Design review of the part built by this model. Coordinates are the model's own, in mm. A direction names the side the tool comes from. Coordinates: 2 decimals unless noted, no trailing zeros. Write each loop counter-clockwise with the first axis right and the second up, starting at its lowest first coordinate (ties: lowest second). Pieces come first, ordered by that corner, then holes. Notation, with made-up numbers: (38, 75) -> (66, 75) arc R19 cw to (66, 100) -> close; hole circle Ø1 at (-17.5, 17.25). An arc over 180 degrees is marked (long way). Answer in a Markdown table with one row per item. Add a question column.
Item 1: Draft analysis for pull direction X (two halves, no side actions). For faces 3 (the face through (7.07, 0.02, 48.13)), 4 (the face through (10, -1.5, 25)), 5 (the face through (-28.6, 0, 26)), state which applies: released by +X, released by -X, zero draft, split by the parting line, or undercut.
Item 2: Take a section at B-B, the plane x = -42.1. Write out the cut boundary in (y, z) (3 decimals).
Item 3: Clearance check with a flat-ended pin moving along its axis: P1, Ø2.5, axis at x = -42.1, z = 5, coming from the +Y side. State where the tip first meets the part, or that it passes through.
Item 4: For faces 1 (the face through (-20.6, 0, 26)), 2 (the face through (50, 0, 59)), list the 3-axis set-ups (+Z, -Z, +X, -X, +Y, -Y) from which the entire face can be reached by the end or side of a thin tool; tool diameter is ignored.
Item 5: Take a section at C-C, the plane z = 41. Give the number of separate pieces and of enclosed holes in the cut face, and give its area (3 significant figures).
Item 6: To check wall thickness, follow line 1 (Z direction, x = 14.5, y = 0.1) (3 decimals); line 2 (X direction, y = 1.25, z = 56.5); line 3 (X direction, y = -1.15, z = -6). State the ranges of each line that lie inside material, in increasing order.
Item 7: Take a section at A-A, the plane x = 27.1. Write out the cut boundary in (y, z) (3 decimals), and give its area (3 significant figures).
from build123d import *

# Parameters (mm, degrees)
EXTRUDE_1_DEPTH      = 55.815
EXTRUDE_1_DEPTH_BACK = 4.185
SKETCH_8_R           = 1.5
CUT_EXTRUDE_1_DEPTH  = 3
SKETCH_11_R          = 1.45
EXTRUDE_4_DEPTH      = 6
EXTRUDE_START        = 6
SKETCH_12_R          = 1.45
EXTRUDE_5_DEPTH      = 6


with BuildPart() as part:
    # 草图1 → 凸台-拉伸1 (new, two sides: drawn at the far end of the back side and taken through both)
    with BuildSketch(Plane.XY.offset(-EXTRUDE_1_DEPTH_BACK)):
        Polygon((50, 0), (50, 1.5), (30, 1.5), (0, 1.5), (-50, 1.5), (-50, -1.5), (30, -1.5), (50, -1.5), align=None)
    extrude(amount=EXTRUDE_1_DEPTH + EXTRUDE_1_DEPTH_BACK)

    # 草图8 → 切除-拉伸1 (cut)
    with BuildSketch(Plane(origin=(0, 1.5, 0), x_dir=(1, 0, 0), z_dir=(0, 1, 0))):
        with BuildLine():
            Line((1.5, -46.63), (1.5, -5))
            ThreePointArc((1.5, -5), (1.060660172, -3.939339828), (0, -3.5))
            ThreePointArc((0, -3.5), (-1.060660172, -3.939339828), (-1.5, -5))
            Line((-1.5, -5), (-1.5, -46.63))
            ThreePointArc((-1.5, -46.63), (0, -48.13), (1.5, -46.63))
        make_face()
        with BuildLine():
            ThreePointArc((-35.6, -5), (-37.1, -3.5), (-38.6, -5))
            Line((-38.6, -5), (-38.6, -46.63))
            ThreePointArc((-38.6, -46.63), (-37.1, -48.13), (-35.6, -46.63))
            Line((-35.6, -46.63), (-35.6, -5))
        make_face()
        with BuildLine():
            ThreePointArc((-30.6, -5), (-32.1, -3.5), (-33.6, -5))
            Line((-33.6, -5), (-33.6, -46.63))
            ThreePointArc((-33.6, -46.63), (-32.1, -48.13), (-30.6, -46.63))
            Line((-30.6, -46.63), (-30.6, -5))
        make_face()
        with BuildLine():
            ThreePointArc((-25.6, -5), (-27.1, -3.5), (-28.6, -5))
            Line((-28.6, -5), (-28.6, -46.63))
            ThreePointArc((-28.6, -46.63), (-27.1, -48.13), (-25.6, -46.63))
            Line((-25.6, -46.63), (-25.6, -5))
        make_face()
        with BuildLine():
            ThreePointArc((-20.6, -5), (-22.1, -3.5), (-23.6, -5))
            Line((-23.6, -5), (-23.6, -46.63))
            ThreePointArc((-23.6, -46.63), (-22.1, -48.13), (-20.6, -46.63))
            Line((-20.6, -46.63), (-20.6, -5))
        make_face()
        with BuildLine():
            ThreePointArc((-15.6, -5), (-17.1, -3.5), (-18.6, -5))
            Line((-18.6, -5), (-18.6, -46.63))
            ThreePointArc((-18.6, -46.63), (-17.1, -48.13), (-15.6, -46.63))
            Line((-15.6, -46.63), (-15.6, -5))
        make_face()
        with BuildLine():
            ThreePointArc((-10.6, -5), (-12.1, -3.5), (-13.6, -5))
            Line((-13.6, -5), (-13.6, -46.63))
            ThreePointArc((-13.6, -46.63), (-12.1, -48.13), (-10.6, -46.63))
            Line((-10.6, -46.63), (-10.6, -5))
        make_face()
        with BuildLine():
            ThreePointArc((-5.6, -5), (-7.1, -3.5), (-8.6, -5))
            Line((-8.6, -5), (-8.6, -46.63))
            ThreePointArc((-8.6, -46.63), (-7.1, -48.13), (-5.6, -46.63))
            Line((-5.6, -46.63), (-5.6, -5))
        make_face()
        with BuildLine():
            ThreePointArc((8.6, -5), (7.1, -3.5), (5.6, -5))
            Line((5.6, -5), (5.6, -46.63))
            ThreePointArc((5.6, -46.63), (7.1, -48.13), (8.6, -46.63))
            Line((8.6, -46.63), (8.6, -5))
        make_face()
        with BuildLine():
            ThreePointArc((13.6, -5), (12.1, -3.5), (10.6, -5))
            Line((10.6, -5), (10.6, -46.63))
            ThreePointArc((10.6, -46.63), (12.1, -48.13), (13.6, -46.63))
            Line((13.6, -46.63), (13.6, -5))
        make_face()
        with BuildLine():
            ThreePointArc((18.6, -5), (17.1, -3.5), (15.6, -5))
            Line((15.6, -5), (15.6, -46.63))
            ThreePointArc((15.6, -46.63), (17.1, -48.13), (18.6, -46.63))
            Line((18.6, -46.63), (18.6, -5))
        make_face()
        with BuildLine():
            ThreePointArc((23.6, -5), (22.1, -3.5), (20.6, -5))
            Line((20.6, -5), (20.6, -46.63))
            ThreePointArc((20.6, -46.63), (22.1, -48.13), (23.6, -46.63))
            Line((23.6, -46.63), (23.6, -5))
        make_face()
        with BuildLine():
            ThreePointArc((28.6, -5), (27.1, -3.5), (25.6, -5))
            Line((25.6, -5), (25.6, -46.63))
            ThreePointArc((25.6, -46.63), (27.1, -48.13), (28.6, -46.63))
            Line((28.6, -46.63), (28.6, -5))
        make_face()
        with BuildLine():
            ThreePointArc((33.6, -5), (32.1, -3.5), (30.6, -5))
            Line((30.6, -5), (30.6, -46.63))
            ThreePointArc((30.6, -46.63), (32.1, -48.13), (33.6, -46.63))
            Line((33.6, -46.63), (33.6, -5))
        make_face()
        with BuildLine():
            ThreePointArc((38.6, -5), (37.1, -3.5), (35.6, -5))
            Line((35.6, -5), (35.6, -46.63))
            ThreePointArc((35.6, -46.63), (37.1, -48.13), (38.6, -46.63))
            Line((38.6, -46.63), (38.6, -5))
        make_face()
        with Locations(Location((-42.1, -5, 0), (0, 0, 270))):
            Circle(SKETCH_8_R)
        with Locations(Location((-42.1, -47.1, 0), (0, 0, 270))):
            Circle(SKETCH_8_R)
        with Locations(Location((42.1, -47.1, 0), (0, 0, 270))):
            Circle(SKETCH_8_R)
        with Locations(Location((42.1, -5, 0), (0, 0, 270))):
            Circle(SKETCH_8_R)
    extrude(amount=-CUT_EXTRUDE_1_DEPTH, mode=Mode.SUBTRACT)

    # 草图11 → 凸台-拉伸4 (add)
    with BuildSketch(Plane.XY.offset(55.815)):
        with Locations(Location((-48.55, 0, 0), (0, 0, 180))):
            Circle(SKETCH_11_R)
        with Locations(Location((48.55, 0, 0), (0, 0, 180))):
            Circle(SKETCH_11_R)
    extrude(amount=EXTRUDE_4_DEPTH)

    # 草图12 → 凸台-拉伸5 (add)
    with BuildSketch(Plane(origin=(0, 0, -4.185), x_dir=(-1, 0, 0), z_dir=(0, 0, -1)).offset(EXTRUDE_START)):
        with Locations((-48.55, 0)):
            Circle(SKETCH_12_R)
        with Locations((48.55, 0)):
            Circle(SKETCH_12_R)
    extrude(amount=-EXTRUDE_5_DEPTH)


solid = part.part
Answers:
| question | item | result |
|---|---|---|
| 1 | face 3 | undercut |
| 1 | face 4 | zero draft |
| 1 | face 5 | undercut |
| 2 | outline | (-1.5, -4.185) -> (1.5, -4.185) -> (1.5, 3.5) -> (-1.5, 3.5) -> close; (-1.5, 6.5) -> (1.5, 6.5) -> (1.5, 45.6) -> (-1.5, 45.6) -> close; (-1.5, 48.6) -> (1.5, 48.6) -> (1.5, 55.815) -> (-1.5, 55.815) -> close |
| 3 | P1 | passes through |
| 4 | face 1 | +Y, -Y |
| 4 | face 2 | +Z |
| 5 | separate pieces | 16 |
| 5 | enclosed holes | 0 |
| 5 | area | 165 mm^2 |
| 6 | line 1 | z = -4.185 to 55.815 |
| 6 | line 2 | x = -49.28 to -47.82, 47.82 to 49.28 |
| 6 | line 3 | x = -49.43 to -47.67, 47.67 to 49.43 |
| 7 | outline | (-1.5, -4.185) -> (1.5, -4.185) -> (1.5, 3.5) -> (-1.5, 3.5) -> close; (-1.5, 48.13) -> (1.5, 48.13) -> (1.5, 55.815) -> (-1.5, 55.815) -> close |
| 7 | area | 46.1 mm^2 |
